from build123d import *

# Parameters (mm, degrees)
SKETCH_1_R          = 9
EXTRUDE_1_DEPTH     = 5
SKETCH_2_R          = 2
CUT_EXTRUDE_1_DEPTH = 5
CHAMFER_1_SIZE      = 1
SKETCH_3_W          = 2
SKETCH_3_H          = 0.5
CUT_EXTRUDE_2_DEPTH = 7


with BuildPart() as part:
    # 草图1 → 凸台-拉伸1 (new body)
    with BuildSketch(Plane.XY):
        with BuildLine():
            Line((37.5, 34.687288473), (37.5, 9.687288473))
            Line((37.5, 9.687288473), (77.5, 9.687288473))
            ThreePointArc((77.5, 9.687288473), (85, 2.187288473), (77.5, -5.312711527))
            Line((77.5, -5.312711527), (11.314817552, -5.312711527))
            ThreePointArc((11.314817552, -5.312711527), (-7.183257499, -10.229897932), (-8.838834765, 8.838834765))
            Line((-8.838834765, 8.838834765), (24.509618943, 42.187288473))
            Line((24.509618943, 42.187288473), (37.5, 34.687288473))
        make_face()
        Circle(SKETCH_1_R, mode=Mode.SUBTRACT)
        with BuildLine():
            Line((77.5, 6.187288473), (32.499999279, 6.187288473))
            ThreePointArc((32.499999279, 6.187288473), (28.5, 2.187288113), (32.5, -1.812711527))
            Line((32.5, -1.812711527), (77.5, -1.812711527))
            ThreePointArc((77.5, -1.812711527), (81.5, 2.187288473), (77.5, 6.187288473))
        make_face(mode=Mode.SUBTRACT)
    extrude(amount=EXTRUDE_1_DEPTH)

    # 草图2 → 切除-拉伸1 (cut)
    with BuildSketch(Plane(origin=(0, 0, 0), x_dir=(-1, 0, 0), z_dir=(0, 0, -1))):
        with Locations((-28.5, 17.687288473)):
            Circle(SKETCH_2_R)
        with Locations((-29.5, 32.38422693)):
            Circle(SKETCH_2_R)
    extrude(amount=-CUT_EXTRUDE_1_DEPTH, mode=Mode.SUBTRACT)

    # 倒角1
    chamfer_1_edges = [part.edges().sort_by_distance(p)[0] for p in [
        (37.5, 9.687288473, 2.5),
    ]]
    chamfer(chamfer_1_edges, length=CHAMFER_1_SIZE)

    # 草图3 → 切除-拉伸2 (cut)
    with BuildSketch(Plane(origin=(0, 0, 0), x_dir=(-1, 0, 0), z_dir=(0, 0, -1))):
        with Locations((-34.343585868, -5.062711527)):
            Rectangle(SKETCH_3_W, SKETCH_3_H)
    extrude(amount=-CUT_EXTRUDE_2_DEPTH, mode=Mode.SUBTRACT)


solid = part.part
Build history of the part. All positions in model axes, mm. A direction names the side the tool comes from. Round coordinates to 2 decimals unless told otherwise and drop trailing zeros. Write each loop counter-clockwise with the first axis right and the second up, starting at its lowest first coordinate (ties: lowest second). Pieces come first, ordered by that corner, then holes. Notation, with made-up numbers: (26.5, 57.5) -> (69.5, 57.5) arc R22 ccw to (69.5, 75.5) -> close; hole circle Ø6 at (-7, 32.25). An arc over 180 degrees is marked (long way). Write item = value, one per line.
(1) Flat gauge pins, fed straight in: pin 1 (1.5 mm diameter, centred on y = 30, z = 1.5, fed in from -X); pin 2 (1.5 mm diameter, centred on y = 2.5, z = 1.5, fed in from +X); pin 3 (3 mm diameter, centred on x = 28.5, y = 17.69, fed in from -Z); pin 4 (2 mm diameter, centred on y = 6, z = 1, fed in from +X). Where does each tip first touch, or does it go through?
Answer:
pin_1 = 11.57
pin_2 = 85
pin_3 = through
pin_4 = 84.45
(2) Band-saw the part on D-D (z = 1.15). Give the cut face in (x, y).
Answer:
outline = (-8.84, 8.84) arc R12.5 ccw (long way) to (11.31, -5.31) -> (33.34, -5.31) -> (33.34, -4.81) -> (35.34, -4.81) -> (35.34, -5.31) -> (77.5, -5.31) arc R7.5 ccw to (77.5, 9.69) -> (38.5, 9.69) -> (37.5, 10.69) -> (37.5, 34.69) -> (24.51, 42.19) -> close; hole circle Ø18 at (0, 0); hole circle Ø4 at (28.5, 17.69); hole circle Ø4 at (29.5, 32.38); hole (32.5, -1.81) -> (77.5, -1.81) arc R4 ccw to (77.5, 6.19) -> (32.5, 6.19) arc R4 ccw to start
(3) Band-saw the part on B-B (y = -3). Give the cut face in (x, z), then the cut area to 3 significant figures.
Answer:
outline = (-12.13, 0) -> (-8.49, 0) -> (-8.49, 5) -> (-12.13, 5) -> close; (8.49, 0) -> (82.92, 0) -> (82.92, 5) -> (8.49, 5) -> close
area = 390 mm2
(4) Probe L1, parallel to Y at x = 41, z = 1.6; L2, parallel to Y at x = 29, z = 3.05; L3, parallel to X at y = 4, z = 4.25. List the from-to ranges inside material, lowest first.
Answer:
L1 = -5.31 to -1.81, 6.19 to 9.69
L2 = -5.31 to 0.25, 4.12 to 15.75, 19.62 to 30.45, 34.32 to 39.59
L3 = -11.84 to -8.06, 8.06 to 28.93, 81.07 to 84.78
(5) Band-saw the part on C-C (x = 29.5). Give the cut face in (y, z), then the cut area to 3 significant figures.
Answer:
outline = (-5.31, 0) -> (-0.46, 0) -> (-0.46, 5) -> (-5.31, 5) -> close; (4.83, 0) -> (15.96, 0) -> (15.96, 5) -> (4.83, 5) -> close; (19.42, 0) -> (30.38, 0) -> (30.38, 5) -> (19.42, 5) -> close; (34.38, 0) -> (39.31, 0) -> (39.31, 5) -> (34.38, 5) -> close
area = 159 mm2
(6) Band-saw the part on A-A (x = 68). Give the cut face in (y, z), then the cut area to 3 significant figures.
Answer:
outline = (-5.31, 0) -> (-1.81, 0) -> (-1.81, 5) -> (-5.31, 5) -> close; (6.19, 0) -> (9.69, 0) -> (9.69, 5) -> (6.19, 5) -> close
area = 35.0 mm2
(7) Tool access for faces 5 (the face through (57, -5.313, 2)), 6 (the face through (55, -1.813, 2)), 7 (the face through (58, 9.687, 2)): list every direction of +Z, -Z, +X, -X, +Y, -Y with a clear straight run to the whole face (end or side of a thin tool).
Answer:
face_5 = +Z, -Z, +X, -Y
face_6 = +Z, -Z
face_7 = +Z, -Z, +X, +Y
(8) Two-plate mould, pull along Y, no slides. Class faces 1 (the face through (28.5, 2.3, 2.5)), 2 (the face through (-6.931, -10.402, 2.465)), 3 (the face through (37.5, 23, 2)), 4 (the face through (34, -4.813, 2)): pulls with the +Y half, pulls with the -Y half, needs draft (parallel to the pull), parting line crosses it, or undercut.
Answer:
face_1 = undercut
face_2 = parting line crosses it
face_3 = needs draft
face_4 = pulls with the -Y half
